Can you work these out from the model? Positions are in its coordinate system, mm. A direction names the side the tool comes from. Coordinates: 2 decimals unless noted, no trailing zeros. Order: outer loops, then holes, each group sorted by start corner. A loop starts at its lowest first (then second) coordinate and runs counter-clockwise, first axis right, second up.
```python
from build123d import *
from OCP.BRepFilletAPI import BRepFilletAPI_MakeChamfer

# Parameters (mm, degrees)
SKETCH2_W                     = 1.5
SKETCH2_H                     = 0.813085377
CUT_EXTRUDE1_DEPTH            = 8
CHAMFER1_SIZE                 = 4
CHAMFER1_SIZE2                = 0.349954654
CIRPATTERN1_COUNT             = 5
CHAMFER1_OF_CIRPATTERN1_SIZE  = 4
CHAMFER1_OF_CIRPATTERN1_SIZE2 = 0.349954654


with BuildPart() as part:
    # Sketch1 → Revolve1 (revolve)
    with BuildSketch(Plane(origin=(0, 0, 0), x_dir=(0, 0, -1), z_dir=(1, 0, 0)), mode=Mode.PRIVATE) as revolve1_sk:
        Polygon((21.5, -20), (21.5, 0), (29.164360148, 0), (29.5, -0.4), (26.1, -1.4), (26.1, -0.4), (22.3, -0.4), (22.3, -20), align=None)
    revolve(revolve1_sk.sketch.rotate(Axis((0, 64.33779776, 0), (0, -1, 0)), 180), axis=Axis((0, 64.33779776, 0), (0, -1, 0)))

    # Sketch2 → Cut-Extrude1 (cut)
    with BuildSketch(Plane.XZ.offset(20)):
        with Locations((0, 21.893457312)):
            Rectangle(SKETCH2_W, SKETCH2_H)
    cut_extrude1 = extrude(amount=-CUT_EXTRUDE1_DEPTH, mode=Mode.SUBTRACT)

    # Chamfer1: one chamfer whose edges measure the first distance from different faces: ONE call of the kernel's chamfer builder (chamfer() names one face for all edges)
    chamfer1_edges_1 = [part.edges().sort_by_distance(p)[0] for p in [
        (-0.75, -20, 21.887149473),
    ]]
    chamfer1_side_1 = [part.faces().sort_by_distance(p)[0] for p in [
        (-0.75, -16, 21.887149473),
    ]]
    chamfer1_edges_2 = [part.edges().sort_by_distance(p)[0] for p in [
        (0.75, -20, 21.887149473),
    ]]
    chamfer1_side_2 = [part.faces().sort_by_distance(p)[0] for p in [
        (0.75, -16, 21.887149473),
    ]]
    chamfer1 = BRepFilletAPI_MakeChamfer(part.part.solid().wrapped)
    for e in chamfer1_edges_1:
        chamfer1.Add(CHAMFER1_SIZE, CHAMFER1_SIZE2, e.wrapped, chamfer1_side_1[0].wrapped)  # the first distance lies on this face
    for e in chamfer1_edges_2:
        chamfer1.Add(CHAMFER1_SIZE, CHAMFER1_SIZE2, e.wrapped, chamfer1_side_2[0].wrapped)  # the first distance lies on this face
    add(Compound.cast(chamfer1.Shape()), mode=Mode.REPLACE)

    # CirPattern1: Cut-Extrude1 ×5 about axis
    cirpattern1_axis = Axis((0, 0, 0), (0, 1, 0))
    for i in range(1, CIRPATTERN1_COUNT):
        add(cut_extrude1.rotate(cirpattern1_axis, i * 360 / CIRPATTERN1_COUNT), mode=Mode.SUBTRACT)

    # Chamfer1 of CirPattern1: one chamfer whose edges measure the first distance from different faces: ONE call of the kernel's chamfer builder (chamfer() names one face for all edges)
    chamfer1_of_cirpattern1_edges_1 = [part.edges().sort_by_distance(p)[0] for p in [
        (20.584153384, -20, 7.476793533),
    ]]
    chamfer1_of_cirpattern1_side_1 = [part.faces().sort_by_distance(p)[0] for p in [
        (20.584153384, -16, 7.476793533),
    ]]
    chamfer1_of_cirpattern1_edges_2 = [part.edges().sort_by_distance(p)[0] for p in [
        (21.047678875, -20, 6.050208758),
    ]]
    chamfer1_of_cirpattern1_side_2 = [part.faces().sort_by_distance(p)[0] for p in [
        (21.047678875, -16, 6.050208758),
    ]]
    chamfer1_of_cirpattern1_edges_3 = [part.edges().sort_by_distance(p)[0] for p in [
        (13.471706421, -20, -17.266236943),
    ]]
    chamfer1_of_cirpattern1_side_3 = [part.faces().sort_by_distance(p)[0] for p in [
        (13.471706421, -16, -17.266236943),
    ]]
    chamfer1_of_cirpattern1_edges_4 = [part.edges().sort_by_distance(p)[0] for p in [
        (12.258180929, -20, -18.147914822),
    ]]
    chamfer1_of_cirpattern1_side_4 = [part.faces().sort_by_distance(p)[0] for p in [
        (12.258180929, -16, -18.147914822),
    ]]
    chamfer1_of_cirpattern1_edges_5 = [part.edges().sort_by_distance(p)[0] for p in [
        (-12.258180929, -20, -18.147914822),
    ]]
    chamfer1_of_cirpattern1_side_5 = [part.faces().sort_by_distance(p)[0] for p in [
        (-12.258180929, -16, -18.147914822),
    ]]
    chamfer1_of_cirpattern1_edges_6 = [part.edges().sort_by_distance(p)[0] for p in [
        (-13.471706421, -20, -17.266236943),
    ]]
    chamfer1_of_cirpattern1_side_6 = [part.faces().sort_by_distance(p)[0] for p in [
        (-13.471706421, -16, -17.266236943),
    ]]
    chamfer1_of_cirpattern1_edges_7 = [part.edges().sort_by_distance(p)[0] for p in [
        (-21.047678875, -20, 6.050208758),
    ]]
    chamfer1_of_cirpattern1_side_7 = [part.faces().sort_by_distance(p)[0] for p in [
        (-21.047678875, -16, 6.050208758),
    ]]
    chamfer1_of_cirpattern1_edges_8 = [part.edges().sort_by_distance(p)[0] for p in [
        (-20.584153384, -20, 7.476793533),
    ]]
    chamfer1_of_cirpattern1_side_8 = [part.faces().sort_by_distance(p)[0] for p in [
        (-20.584153384, -16, 7.476793533),
    ]]
    chamfer1_of_cirpattern1 = BRepFilletAPI_MakeChamfer(part.part.solid().wrapped)
    for e in chamfer1_of_cirpattern1_edges_1:
        chamfer1_of_cirpattern1.Add(CHAMFER1_OF_CIRPATTERN1_SIZE, CHAMFER1_OF_CIRPATTERN1_SIZE2, e.wrapped, chamfer1_of_cirpattern1_side_1[0].wrapped)  # the first distance lies on this face
    for e in chamfer1_of_cirpattern1_edges_2:
        chamfer1_of_cirpattern1.Add(CHAMFER1_OF_CIRPATTERN1_SIZE, CHAMFER1_OF_CIRPATTERN1_SIZE2, e.wrapped, chamfer1_of_cirpattern1_side_2[0].wrapped)  # the first distance lies on this face
    for e in chamfer1_of_cirpattern1_edges_3:
        chamfer1_of_cirpattern1.Add(CHAMFER1_OF_CIRPATTERN1_SIZE, CHAMFER1_OF_CIRPATTERN1_SIZE2, e.wrapped, chamfer1_of_cirpattern1_side_3[0].wrapped)  # the first distance lies on this face
    for e in chamfer1_of_cirpattern1_edges_4:
        chamfer1_of_cirpattern1.Add(CHAMFER1_OF_CIRPATTERN1_SIZE, CHAMFER1_OF_CIRPATTERN1_SIZE2, e.wrapped, chamfer1_of_cirpattern1_side_4[0].wrapped)  # the first distance lies on this face
    for e in chamfer1_of_cirpattern1_edges_5:
        chamfer1_of_cirpattern1.Add(CHAMFER1_OF_CIRPATTERN1_SIZE, CHAMFER1_OF_CIRPATTERN1_SIZE2, e.wrapped, chamfer1_of_cirpattern1_side_5[0].wrapped)  # the first distance lies on this face
    for e in chamfer1_of_cirpattern1_edges_6:
        chamfer1_of_cirpattern1.Add(CHAMFER1_OF_CIRPATTERN1_SIZE, CHAMFER1_OF_CIRPATTERN1_SIZE2, e.wrapped, chamfer1_of_cirpattern1_side_6[0].wrapped)  # the first distance lies on this face
    for e in chamfer1_of_cirpattern1_edges_7:
        chamfer1_of_cirpattern1.Add(CHAMFER1_OF_CIRPATTERN1_SIZE, CHAMFER1_OF_CIRPATTERN1_SIZE2, e.wrapped, chamfer1_of_cirpattern1_side_7[0].wrapped)  # the first distance lies on this face
    for e in chamfer1_of_cirpattern1_edges_8:
        chamfer1_of_cirpattern1.Add(CHAMFER1_OF_CIRPATTERN1_SIZE, CHAMFER1_OF_CIRPATTERN1_SIZE2, e.wrapped, chamfer1_of_cirpattern1_side_8[0].wrapped)  # the first distance lies on this face
    add(Compound.cast(chamfer1_of_cirpattern1.Shape()), mode=Mode.REPLACE)


solid = part.part
```
1. Imagine slicing it at A-A on y = -13.5. Please give me the cut outline in (x, z).
Completed:
outline: (-21.43, 6.17) arc R22.3 ccw to (-13.71, -17.59) - (-13.24, -16.94) arc R21.5 cw to (-20.67, 5.93) - close; (-20.96, 7.6) - (-20.2, 7.35) arc R21.5 cw to (-0.75, 21.49) - (-0.75, 22.29) arc R22.3 ccw to start; (-12.49, -18.47) arc R22.3 ccw to (12.49, -18.47) - (12.02, -17.82) arc R21.5 cw to (-12.02, -17.82) - close; (0.75, 21.49) arc R21.5 cw to (20.2, 7.35) - (20.96, 7.6) arc R22.3 ccw to (0.75, 22.29) - close; (13.24, -16.94) - (13.71, -17.59) arc R22.3 ccw to (21.43, 6.17) - (20.67, 5.93) arc R21.5 cw to start
2. Thinking about a two-plate mould opening in Z: for faces 3 (the conical face through (25.64, -1.35, -5.69)), 4 (the flat face through (0, -20, -22)), 5 (the flat face through (-12, -0.4, 19)), 6 (the flat face through (12.9, -12, -17.7)), which applies, pulls with the +Z half, pulls with the -Z half, needs draft (parallel to the pull), parting line crosses it, or undercut?
Completed:
face 3: parting line crosses it
face 4: needs draft
face 5: undercut
face 6: undercut
3. Imagine slicing it at C-C on x = 0. Please give me the cut outline in (y, z).
Completed:
outline: (-20, -22.3) - (-0.4, -22.3) - (-0.4, -26.1) - (-1.4, -26.1) - (-0.4, -29.5) - (0, -29.16) - (0, -21.5) - (-20, -21.5) - close; (-12, 21.5) - (0, 21.5) - (0, 29.16) - (-0.4, 29.5) - (-1.4, 26.1) - (-0.4, 26.1) - (-0.4, 22.3) - (-12, 22.3) - close
4. Imagine slicing it at B-B on z = 0. Please give me the cut outline in (x, y).
Completed:
outline: (-29.5, -0.4) - (-26.1, -1.4) - (-26.1, -0.4) - (-22.3, -0.4) - (-22.3, -20) - (-21.5, -20) - (-21.5, 0) - (-29.16, 0) - close; (21.5, -20) - (22.3, -20) - (22.3, -0.4) - (26.1, -0.4) - (26.1, -1.4) - (29.5, -0.4) - (29.16, 0) - (21.5, 0) - close
5. I'm going to push flat-ended pins straight in: pin 1 (8 mm diameter, centred on x = -20.5, y = -9.5, fed in from -Z); pin 2 (8 mm diameter, centred on x = 4.5, y = -16, fed in from -Z); pin 3 (12 mm diameter, centred on y = -15, z = 18, fed in from -X). Where does each tip first touch, or does it pass through?
Completed:
pin 1: stops at z = -15
pin 2: stops at z = -22.29
pin 3: stops at x = -18.8
6. Please list where these lines run through material, in increasing order: probe 1 along X at (y, z) = (-10.5, 0); probe 2 along Y at (x, z) = (-5, 25.5); probe 3 along Z at (x, y) = (3, -12.75).
Completed:
probe 1: x = -22.3 to -21.5, 21.5 to 22.3
probe 2: y = -0.4 to 0
probe 3: z = -22.1 to -21.29, 21.29 to 22.1
7. Imagine slicing it at D-D on y = -7.75. Please give me the cut outline in (x, z), then the cut area to 3 significant figures.
Completed:
outline: circle Ø44.6 at (0, 0); hole circle Ø43 at (0, 0)
area: 110 mm2
8. On a 3-axis mill with a long thin cutter (end or side, diameter ignored), from which of +Z, -Z, +X, -X, +Y, -Y can I reach the whole of each face in a straight line? I mean faces 1 (the cylindrical face through (-25.878, -0.893, -3.398)), 2 (the flat face through (-11.75, -20, 18.19)). Say none if no direction works.
Completed:
face 1: -Y
face 2: +Z, -Z, +X, -X, -Y
